from build123d import *

# Parameters (mm, degrees)
F0_W     = 44.6
F0_H     = 39.6
F1_DEPTH = 2
F0_W_2   = 22
F0_H_2   = 2
F2_DEPTH = 18
F0_W_3   = 2
F0_H_3   = 20
F3_DEPTH = 23
F4_DEPTH = 3
F5_R     = 1.5
F6_R     = 2


with BuildPart() as f1:
    # F0 (on Top) → F1 (new body)
    with BuildSketch(Plane.XY):
        Polygon((31, 0), (49, 0), (49, 44), (27, 44), (27, 42), (5, 42), (5, 44), (0, 44), (0, 41.8), (0, 41), (2, 41), (2, 21), (0, 21), (0, 0), (9, 0), (9, 2), (31, 2), align=None)
        with Locations((24.5, 22)):
            Rectangle(F0_W, F0_H, mode=Mode.SUBTRACT)
    extrude(amount=-F1_DEPTH)

    # F0 (on Top) → F2 (join)
    with BuildSketch(Plane.XY):
        with Locations((16, 43)):
            Rectangle(F0_W_2, F0_H_2)
        with Locations((20, 1)):
            Rectangle(F0_W_2, F0_H_2)
    extrude(amount=-F2_DEPTH)

    # F0 (on Top) → F3 (join)
    with BuildSketch(Plane.XY):
        with Locations((1, 31)):
            Rectangle(F0_W_3, F0_H_3)
    extrude(amount=-F3_DEPTH)

    # F0 (on Top) → F4 (join)
    with BuildSketch(Plane.XY):
        with Locations((24.5, 22)):
            Rectangle(F0_W, F0_H)
    extrude(amount=-F4_DEPTH)

    # F5
    f5_edges = [f1.edges().sort_by_distance(p)[0] for p in [
        (2.2, 2.2, -2.5),
        (2.2, 41.8, -2.5),
        (46.8, 2.2, -2.5),
        (46.8, 41.8, -2.5),
    ]]
    fillet(f5_edges, radius=F5_R)

    # F6
    f6_edges = [f1.edges().sort_by_distance(p)[0] for p in [
        (5, 43, -18),
        (27, 43, -18),
        (1, 41, -23),
        (1, 21, -23),
        (31, 1, -18),
        (9, 1, -18),
    ]]
    fillet(f6_edges, radius=F6_R)


solid = f1.part
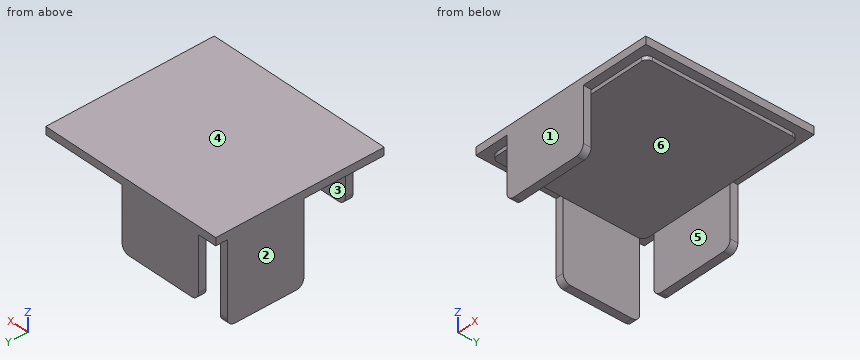
Check sheet for the modelled part. Datum: model origin and axes. Units: mm. Face numbers are marked on the shaded views. A direction names the side the tool comes from. Give positions to 0.01 mm unless a question says otherwise; leave off trailing zeros. Order: outer loops, then holes, each group sorted by start corner. A loop starts at its lowest first (then second) coordinate and runs counter-clockwise, first axis right, second up. Notation, with made-up numbers: M 1,71.25 L 29,71.25 A17 cw 29,88.25 Z; hole C 52.25,-3.5 d8. An arc over 180 degrees is marked long. Answer as CSV lines item,"result". Start each with the question number.
Item 1: Cross-section at A-A on z = -12.75. Enter the section's corners in (x, y), plus the area to 3 significant figures.
Item 2: Tool access check on the marked faces 4, 5 and 6. Record the directions out of +Z, -Z, +X, -X, +Y, -Y that give a thin tool (end or side, any length) a straight path to the whole face; none if there is none.
Item 3: Mould release check, pull along Y, two halves, no side actions. Record for the marked faces 1, 2 and 3: +Y half, -Y half, draft (parallel to the pull), parting line (faces both ways), or undercut.
Item 4: Gauge pin test, flat ends, axial feed: P1, Ø22, axis at x = 22, y = 16.5, coming from the -Z side; P2, Ø1, axis at y = 0.5, z = -7, coming from the +X side; P3, Ø1.6, axis at y = 43.5, z = -10.5, coming from the +X side. Record the tip position at first contact, or that the pin passes through.
Item 5: Cross-section at C-C on x = 3. Enter the section's corners in (y, z), plus the area to 3 significant figures.
Item 6: Cross-section at B-B on y = 16.5. Enter the section's corners in (x, z).
Item 7: Thickness scan on line 1 (Y direction, x = 15, z = -11); line 2 (X direction, y = 25, z = -21.25); line 3 (Z direction, x = 31, y = 2). Record the ranges inside material, lowest first. Write a range as [from, to].
Item 8: Cross-section at D-D on y = 34. Enter the section's corners in (x, z).
Established:
1,outline,"M 0,21 L 2,21 L 2,41 L 0,41 Z; M 5,42 L 27,42 L 27,44 L 5,44 Z; M 9,0 L 31,0 L 31,2 L 9,2 Z"
1,area,"128 mm^2"
2,face 4,"+Z, +X, -X, +Y, -Y"
2,face 5,"-Z, +X, -X"
2,face 6,"-Z, +X"
3,face 1,"-Y half"
3,face 2,"draft"
3,face 3,"undercut"
4,P1,"stops at z = -3"
4,P2,"stops at x = 31"
4,P3,"stops at x = 27"
5,outline,"M 0,-2 L 2.37,-2 L 2.37,-3 L 41.63,-3 L 41.63,-2 L 44,-2 L 44,0 L 0,0 Z"
5,area,"127 mm^2"
6,outline,"M 0,-2 L 2.2,-2 L 2.2,-3 L 46.8,-3 L 46.8,-2 L 49,-2 L 49,0 L 0,0 Z"
7,line 1,"y = [0, 2], [42, 44]"
7,line 2,"x = [0, 2]"
7,line 3,"z = [-2, 0]"
8,outline,"M 0,-23 L 2,-23 L 2,-2 L 2.2,-2 L 2.2,-3 L 46.8,-3 L 46.8,-2 L 49,-2 L 49,0 L 0,0 Z"
